Work out the finished part from the listing and answer in its coordinate system (mm). Face numbers are marked on the shaded views. A direction names the side the tool comes from. Coordinates: 2 decimals unless noted, no trailing zeros. Order: outer loops, then holes, each group sorted by start corner. A loop starts at its lowest first (then second) coordinate and runs counter-clockwise, first axis right, second up. Notation, with made-up numbers: M 56,-26 L 112,-26 A22 cw 112,1 Z; hole C -8,32 d10. An arc over 180 degrees is marked long. Use a Markdown table: item, result.
from build123d import *

# Parameters (mm, degrees)
BOSS_EXTRUDE1_DEPTH     = 50.8
SKETCH3_R               = 8.89
SKETCH3_R_2             = 6.35
CUT_EXTRUDE_THIN1_DEPTH = 7.9375


with BuildPart() as part:
    # Sketch2 → Boss-Extrude1 (new body, symmetric)
    with BuildSketch(Plane(origin=(0, 0, 0), x_dir=(0, 0, -1), z_dir=(1, 0, 0))):
        Polygon((7.332348419, 0), (3.666174209, 6.35), (-3.666174209, 6.35), (-7.332348419, 0), (-3.666174209, -6.35), (3.666174209, -6.35), align=None)
    extrude(amount=BOSS_EXTRUDE1_DEPTH, both=True)

    # Sketch3 → Cut-Extrude-Thin1 (cut)
    with BuildSketch(Plane(origin=(50.8, 0, 0), x_dir=(0, 0, -1), z_dir=(1, 0, 0))):
        Circle(SKETCH3_R)
        Circle(SKETCH3_R_2, mode=Mode.SUBTRACT)
    cut_extrude_thin1 = extrude(amount=-CUT_EXTRUDE_THIN1_DEPTH, mode=Mode.SUBTRACT)

    # Mirror1: Cut-Extrude-Thin1 across plane
    add(cut_extrude_thin1.mirror(Plane(origin=(0, 0, 0), x_dir=(0, 0, 1), z_dir=(1, 0, 0))), mode=Mode.SUBTRACT)


solid = part.part
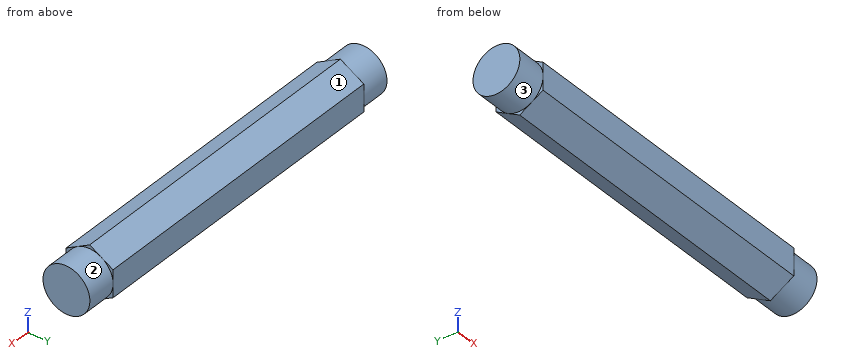
1. For the marked faces 1, 2 and 3, determine the directions among +Z, -Z, +X, -X, +Y, -Y from which every point of the face is accessible in a straight line to the end or side of a thin tool.
Answers below:
| item | result |
|---|---|
| face 1 | +Z, +X, -X, +Y |
| face 2 | +X |
| face 3 | -X |
2. Section A-A on x = -29.5 is taken. Determine the outline of the cut face in (y, z), then the cut area to 3 significant figures.
Answers below:
| item | result |
|---|---|
| outline | M -6.35,-3.67 L 0,-7.33 L 6.35,-3.67 L 6.35,3.67 L 0,7.33 L -6.35,3.67 Z |
| area | 140 mm² |
3. Section B-B on z = -4.5 is taken. Determine the outline of the cut face in (x, y), then the cut area to 3 significant figures.
Answers below:
| item | result |
|---|---|
| outline | M -50.8,-4.48 L -42.86,-4.48 L -42.86,-4.91 L 42.86,-4.91 L 42.86,-4.48 L 50.8,-4.48 L 50.8,4.48 L 42.86,4.48 L 42.86,4.91 L -42.86,4.91 L -42.86,4.48 L -50.8,4.48 Z |
| area | 983 mm² |
4. Find the intervals of material crossed by probe 1 along Y at (x, z) = (17, -5.5); probe 2 along X at (y, z) = (-5.5, 3.75); probe 3 along Y at (x, z) = (27, -3.75), in increasing order.
Answers below:
| item | result |
|---|---|
| probe 1 | -3.17 to 3.17 |
| probe 2 | -42.86 to 42.86 |
| probe 3 | -6.2 to 6.2 |
5. Flat-ended cylindrical pins translate along their axes: P1, Ø2.5, axis at y = 5.5, z = 4, coming from the -X side; P2, Ø4, axis at x = 19.5, y = 4, coming from the -Z side; P3, Ø1, axis at x = -17, y = 4, coming from the -Z side. Find the tip coordinate at first contact, or state that the pin passes through.
Answers below:
| item | result |
|---|---|
| P1 | x = -50.8 |
| P2 | z = -6.18 |
| P3 | z = -5.31 |
